The figure shows three views and two pictorial views of one solid part (mm, origin at its lowest corner). Answer the questions. A direction names the side the tool comes from. Round coordinates to 2 decimals unless told otherwise and drop trailing zeros. Order: outer loops, then holes, each group sorted by start corner. A loop starts at its lowest first (then second) coordinate and runs counter-clockwise, first axis right, second up. Notation, with made-up numbers: (48.5, 63) - (88.5, 63) arc R26 cw to (88.5, 80) - close; hole circle Ø4 at (16, 44.25). An arc over 180 degrees is marked (long way). One line per item, written item: value. Start each with the question number.
1. Section A-A, the plane x = 25 is taken. Give the vertices of the cut face in (y, z), then the cut area to 3 significant figures.
2. A tool of negligible diameter and unlimited length cuts with its end or side. For the marked faces 1, 2 and 3, from which of +Z, -Z, +X, -X, +Y, -Y can it reach the whole face along a straight path? Write none if from no direction.
3. Section B-B, the plane z = 25 is taken. Give the vertices of the cut face in (x, y), then the cut area to 3 significant figures.
4. Flat-ended cylindrical pins translate along their axes: P1, Ø10, axis at x = 32, z = 105, coming from the +Y side; P2, Ø5, axis at x = 40, y = 25, coming from the -Z side; P3, Ø22, axis at x = 36, y = 11, coming from the -Z side. Find the tip coordinate at first contact, or state that the pin passes through.
5. Straight lines are drawn through the part: line 1 (X direction, y = 35, z = 25); line 2 (Z direction, x = 26, y = 35); line 3 (Y direction, x = 45, z = 139). For each, find the intervals that lie inside material, in ascending order.
6. Section C-C, the plane x = 8.5 is taken. Give the vertices of the cut face in (y, z), then the cut area to 3 significant figures.
7. Section D-D, the plane z = 202 is taken. Give the vertices of the cut face in (x, y), then the cut area to 3 significant figures.
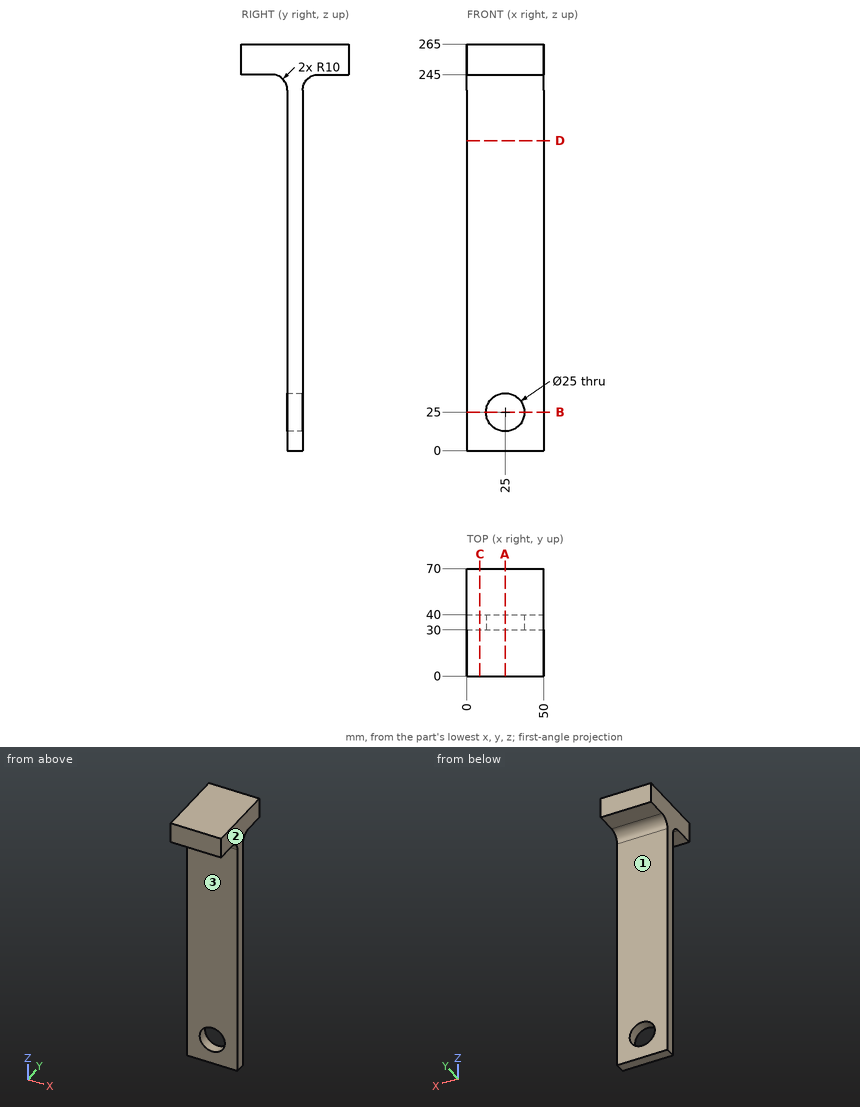
Answer list:
1. outline: (0, 245) - (20, 245) arc R10 cw to (30, 235) - (30, 37.5) - (40, 37.5) - (40, 235) arc R10 cw to (50, 245) - (70, 245) - (70, 265) - (0, 265) - close; (30, 0) - (40, 0) - (40, 12.5) - (30, 12.5) - close
1. area: 3,640 mm²
2. face 1: -Z, +X, -X, +Y
2. face 2: +Z, -Z, +X, +Y, -Y
2. face 3: -Z, +X, -X, -Y
3. outline: (0, 30) - (12.5, 30) - (12.5, 40) - (0, 40) - close; (37.5, 30) - (50, 30) - (50, 40) - (37.5, 40) - close
3. area: 250 mm²
4. P1: stops at y = 40
4. P2: stops at z = 241.61
4. P3: stops at z = 244.8
5. line 1: x = 0 to 12.5, 37.5 to 50
5. line 2: z = 0 to 12.54, 37.46 to 265
5. line 3: y = 30 to 40
6. outline: (0, 245) - (20, 245) arc R10 cw to (30, 235) - (30, 0) - (40, 0) - (40, 235) arc R10 cw to (50, 245) - (70, 245) - (70, 265) - (0, 265) - close
6. area: 3,890 mm²
7. outline: (0, 30) - (50, 30) - (50, 40) - (0, 40) - close
7. area: 500 mm²
